from build123d import *

# Parameters (mm, degrees)
F1_DEPTH = 2


with BuildPart() as f1:
    # F0 (on Front) → F1 (new body)
    with BuildSketch(Plane.XZ):
        Polygon((-31.935285, 51.427654), (-54.041285, 70.032309), (-84.041285, 44.783976), (-102.041285, 11.482309), (-31.935285, 11.482309), align=None)
        Polygon((-56.541285, 16.482309), (-93.655068, 16.482309), (-80.094596, 41.570438), (-56.541285, 61.393166), align=None, mode=Mode.SUBTRACT)
        Polygon((-36.935285, 49.100595), (-36.935285, 16.482309), (-51.541285, 16.482309), (-51.541285, 61.393166), align=None, mode=Mode.SUBTRACT)
    extrude(amount=F1_DEPTH)


solid = f1.part
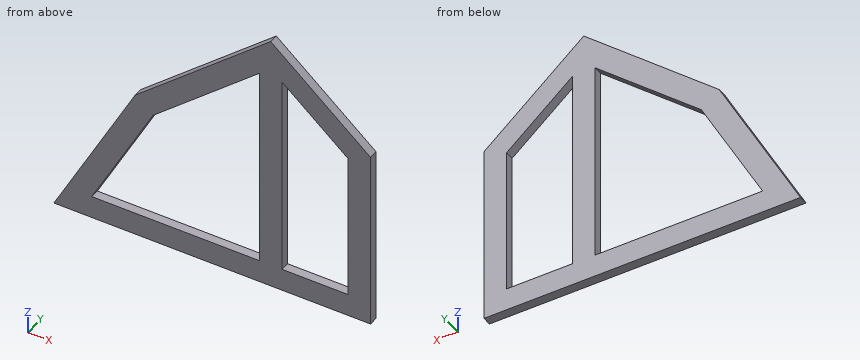
Input: part model. Units: mm. Frame: model coordinates. Coordinates: 2 decimals unless noted, no trailing zeros. Loops run counter-clockwise (first coordinate to the right, second up) from the corner with the lowest first, then second, coordinate; pieces in that order, holes last. Notation, with made-up numbers: (87.5, 40.5) -> (108.5, 40.5) arc R18 cw to (108.5, 61.5) -> close; hole circle Ø8 at (80.25, 72.25). An arc over 180 degrees is marked (long way). Write item = value, one per line. Start each with the question number.
Item 1: Cut plane A-A, the plane y = -1.7. Return loops of the section in (x, z), plus the area to 3 significant figures.
Item 2: Material intervals for line 1 (X direction, y = -0.4, z = 18.5); line 2 (X direction, y = -0.3, z = 20.5); line 3 (Z direction, x = -74, y = -1.8), sorted ascending.
Item 3: Cut plane C-C, the plane x = -68.5. Return loops of the section in (y, z).
Item 4: First-contact query: P1, Ø0.6, axis at x = -83, y = -1, coming from the +Z side; P2, Ø1, axis at y = -0.5, z = 31.5, coming from the -X side; P3, Ø1, axis at x = -45.5, y = -1.5, coming from the +Z side. Flat tips, straight axial feed; report the tip coordinate or a pass-through.
Item 5: Cut plane B-B, the plane z = 42.5. Return loops of the section in (x, y), plus the area to 3 significant figures.
Item 6: Cut plane D-D, the plane z = 60.5. Return loops of the section in (x, y).
Ans:
q1.outline = (-102.04, 11.48) -> (-31.94, 11.48) -> (-31.94, 51.43) -> (-54.04, 70.03) -> (-84.04, 44.78) -> close; hole (-93.66, 16.48) -> (-56.54, 16.48) -> (-56.54, 61.39) -> (-80.09, 41.57) -> close; hole (-51.54, 16.48) -> (-36.94, 16.48) -> (-36.94, 49.1) -> (-51.54, 61.39) -> close
q1.area = 1,210 mm²
q2.line_1 = -98.25 to -92.56, -56.54 to -51.54, -36.94 to -31.94
q2.line_2 = -97.17 to -91.48, -56.54 to -51.54, -36.94 to -31.94
q2.line_3 = 11.48 to 16.48, 46.7 to 53.23
q3.outline = (-2, 11.48) -> (0, 11.48) -> (0, 16.48) -> (-2, 16.48) -> close; (-2, 51.33) -> (0, 51.33) -> (0, 57.86) -> (-2, 57.86) -> close
q4.P1 = 45.91
q4.P2 = -91.49
q4.P3 = 63.26
q5.outline = (-85.28, -2) -> (-78.99, -2) -> (-78.99, 0) -> (-85.28, 0) -> close; (-56.54, -2) -> (-51.54, -2) -> (-51.54, 0) -> (-56.54, 0) -> close; (-36.94, -2) -> (-31.94, -2) -> (-31.94, 0) -> (-36.94, 0) -> close
q5.area = 32.6 mm²
q6.outline = (-65.37, -2) -> (-57.6, -2) -> (-57.6, 0) -> (-65.37, 0) -> close; (-56.54, -2) -> (-51.54, -2) -> (-51.54, 0) -> (-56.54, 0) -> close; (-50.48, -2) -> (-42.72, -2) -> (-42.72, 0) -> (-50.48, 0) -> close
